Geometry: see drawing. Coordinates: mm, zero at the bounding-box minimum. A direction names the side the tool comes from. Round coordinates to 2 decimals unless told otherwise and drop trailing zeros. Write each loop counter-clockwise with the first axis right and the second up, starting at its lowest first coordinate (ties: lowest second). Pieces come first, ordered by that corner, then holes. Notation, with made-up numbers: M 27,17 L 73,17 A10 cw 73,21 Z; hole C 25,58.5 d9. An arc over 180 degrees is marked long. Use a Markdown table: item, result.
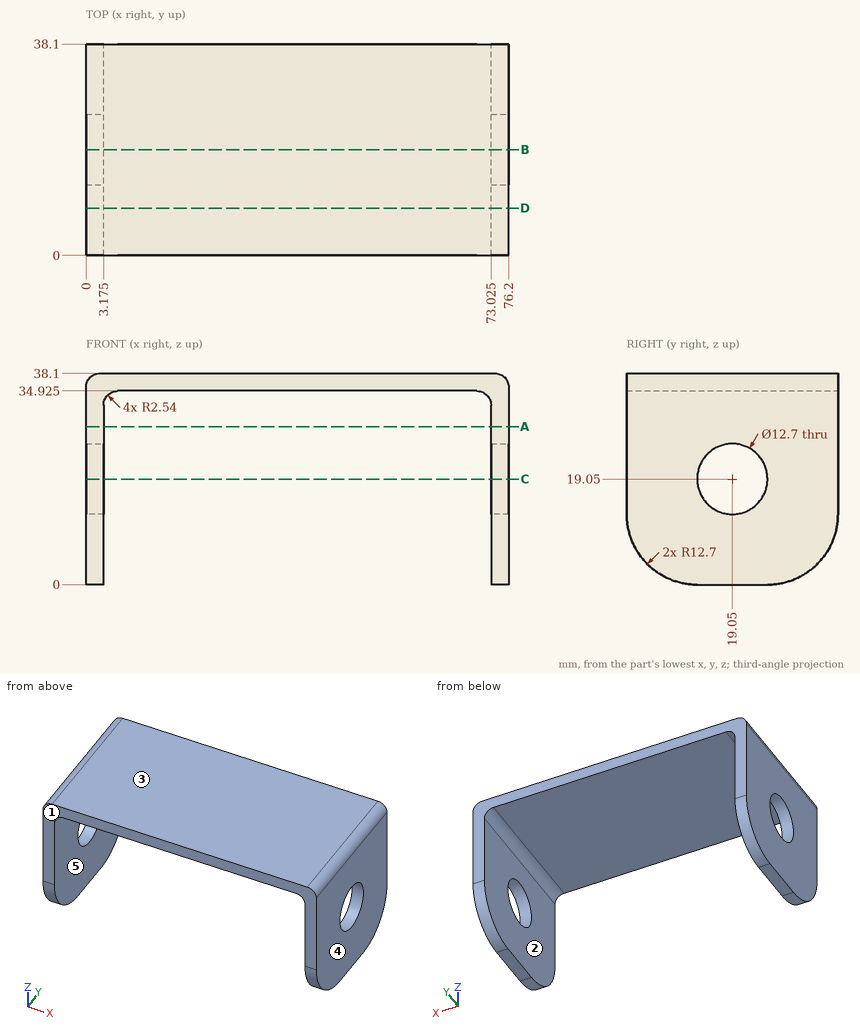
Q1. Mould query, pull axis X, two halves, no side actions, for the marked faces 3, 4 and 5. Classes: +X half, -X half, draft (parallel to the pull), parting line (faces both ways), or undercut.
Results are:
| item | result |
|---|---|
| face 3 | draft |
| face 4 | +X half |
| face 5 | undercut |
Q2. Section C-C on z = 19.05. Return loops of the section in (x, y) (3 decimals).
Results are:
| item | result |
|---|---|
| outline | M 0,0 L 3.175,0 L 3.175,12.7 L 0,12.7 Z; M 0,25.4 L 3.175,25.4 L 3.175,38.1 L 0,38.1 Z; M 73.025,0 L 76.2,0 L 76.2,12.7 L 73.025,12.7 Z; M 73.025,25.4 L 76.2,25.4 L 76.2,38.1 L 73.025,38.1 Z |
Q3. Section B-B on y = 19.05. Return loops of the section in (x, z) (3 decimals), plus the area to 3 significant figures.
Results are:
| item | result |
|---|---|
| outline | M 0,0 L 3.175,0 L 3.175,12.7 L 0,12.7 Z; M 0,25.4 L 3.175,25.4 L 3.175,32.385 A2.54 cw 5.715,34.925 L 70.485,34.925 A2.54 cw 73.025,32.385 L 73.025,25.4 L 76.2,25.4 L 76.2,35.56 A2.54 ccw 73.66,38.1 L 2.54,38.1 A2.54 ccw 0,35.56 Z; M 73.025,0 L 76.2,0 L 76.2,12.7 L 73.025,12.7 Z |
| area | 383 mm^2 |
Q4. First-contact query: pin 1 Ø10 at (y, z) = (19.05, 19.05) entering from -X; pin 2 Ø12 at (x, y) = (14, 14) entering from -Z (3 decimals). Flat tips, straight axial feed; report the tip coordinate or a pass-through.
Results are:
| item | result |
|---|---|
| pin 1 | through |
| pin 2 | z = 34.925 |
Q5. Line query: L1, parallel to X at y = 26.5, z = 14 (3 decimals); L2, parallel to Y at x = 75.3, z = 19.05; L3, parallel to Z at x = 39, y = 32.5 (3 decimals). Output: solid intervals per line, ascending.
Results are:
| item | result |
|---|---|
| L1 | 0 to 3.175, 73.025 to 76.2 |
| L2 | 0 to 12.7, 25.4 to 38.1 |
| L3 | 34.925 to 38.1 |
Q6. Section A-A on z = 28.5. Return loops of the section in (x, y) (3 decimals), plus the area to 3 significant figures.
Results are:
| item | result |
|---|---|
| outline | M 0,0 L 3.175,0 L 3.175,38.1 L 0,38.1 Z; M 73.025,0 L 76.2,0 L 76.2,38.1 L 73.025,38.1 Z |
| area | 242 mm^2 |
Q7. Section D-D on y = 8.5. Return loops of the section in (x, z) (3 decimals), plus the area to 3 significant figures.
Results are:
| item | result |
|---|---|
| outline | M 0,0.715 L 3.175,0.715 L 3.175,32.385 A2.54 cw 5.715,34.925 L 70.485,34.925 A2.54 cw 73.025,32.385 L 73.025,0.715 L 76.2,0.715 L 76.2,35.56 A2.54 ccw 73.66,38.1 L 2.54,38.1 A2.54 ccw 0,35.56 Z |
| area | 459 mm^2 |
Q8. Reachability of the marked faces 1 and 2 from +Z, -Z, +X, -X, +Y, -Y: full face, straight path, thin tool, end or side. Return the list, or none.
Results are:
| item | result |
|---|---|
| face 1 | +Z, -Z, +X, -X, -Y |
| face 2 | -Z, +Y, -Y |
